Could you check a few things on this drawing? It's one solid part, dimensions in mm from its lowest x, y, z. A direction names the side the tool comes from. Give positions to 0.01 mm unless a question says otherwise; leave off trailing zeros. Loops run counter-clockwise (first coordinate to the right, second up) from the corner with the lowest first, then second, coordinate; pieces in that order, holes last. Notation, with made-up numbers: M 57,-29.75 L 75,-29.75 A18 cw 75,-13.75 Z; hole C 77,-39 d5. An arc over 180 degrees is marked long. Answer as CSV lines item,"result". Start each with the question number.
Item 1: If I drill on line 1 along X through (y, z) = (49, 3.5); line 2 along X through (y, z) = (20, 29.5); line 3 along X through (y, z) = (6.5, 3), over which ranges is the centre line in solid material (lowest first)? Write a range as from..to.
Item 2: For the marked faces 1, 2, 3, 4 and 5, which set-ups out of +Z, -Z, +X, -X, +Y, -Y let a thin tool reach every point of the face, with its end or its side?
Item 3: Will these pins go through, and if not, where does the flat tip stop? P1, Ø3, axis at y = 30.5, z = 32, coming from the +X side; P2, Ø0.8, axis at x = 32.5, z = 67, coming from the -Y side; P3, Ø3, axis at x = 39.45, z = 37.92, coming from the -Y side; P4, Ø1.5, axis at y = 33.5, z = 41.5, coming from the -X side.
Item 4: If we mould it in two halves opening along Z, with no side actions, what happens to the marked faces 6, 7 and 8? For each: released by +Z, released by -Z, zero draft, split by the parting line, or undercut.
Item 5: I want a section at B-B on z = 35. List the corners of the cut face in (x, y) for me.
Item 6: I want a section at A-A on x = 33. List the corners of the cut face in (y, z) for me, plus the area to 3 significant figures.
Item 7: I want a section at C-C on x = 45.5. List the corners of the cut face in (y, z) for me.
Item 8: I want a section at D-D on y = 26. List the corners of the cut face in (x, z) for me.
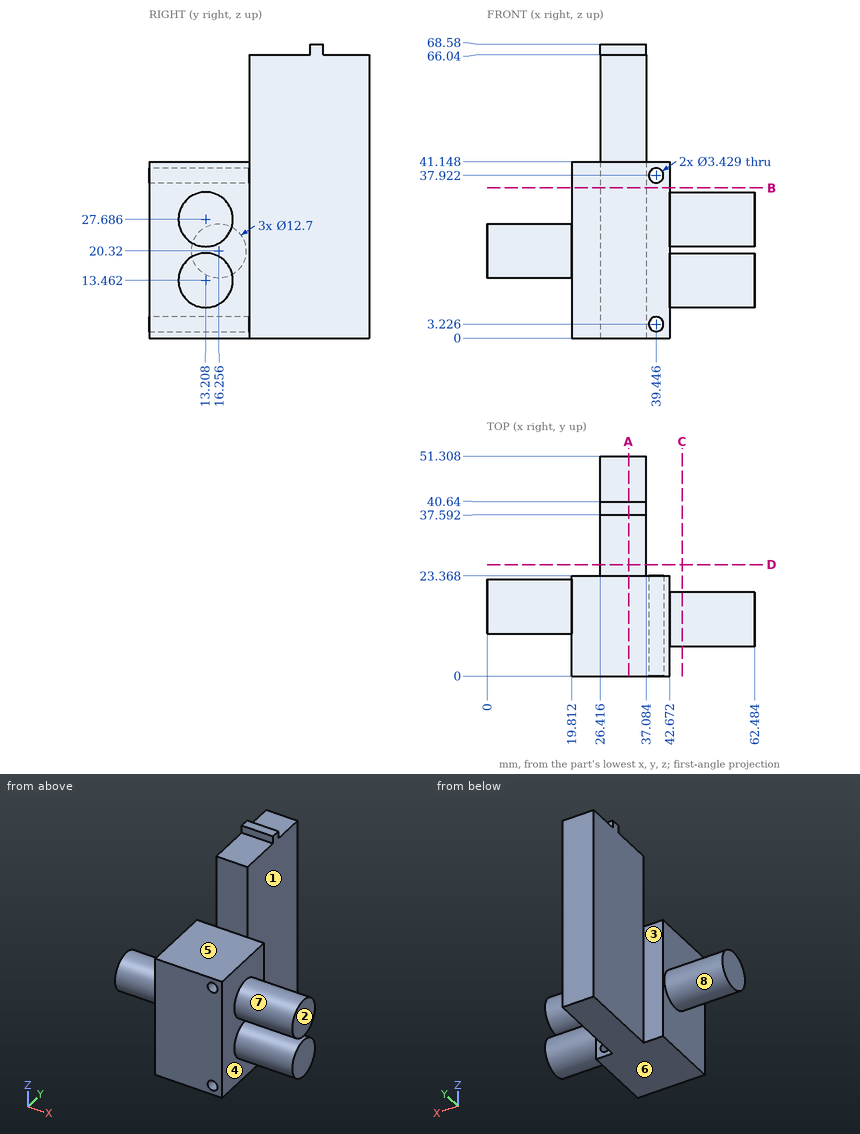
Result:
1,line 1,"26.42..37.08"
1,line 2,"19.81..42.67"
1,line 3,"19.81..37.75, 41.15..42.67"
2,face 1,"+Z, -Z, +X, +Y"
2,face 2,"+Z, -Z, +X, +Y, -Y"
2,face 3,"+Z, -Z, -X, +Y"
2,face 4,"+X"
2,face 5,"+Z, +X, -X, -Y"
3,P1,"x = 37.08"
3,P2,"y = 37.59"
3,P3,"through"
3,P4,"x = 26.42"
4,face 6,"released by -Z"
4,face 7,"undercut"
4,face 8,"split by the parting line"
5,outline,"M 19.81,0 L 42.67,0 L 42.67,23.37 L 37.08,23.37 L 37.08,51.31 L 26.42,51.31 L 26.42,23.37 L 19.81,23.37 Z"
6,outline,"M 0,0 L 51.31,0 L 51.31,66.04 L 40.64,66.04 L 40.64,68.58 L 37.59,68.58 L 37.59,66.04 L 23.37,66.04 L 23.37,41.15 L 0,41.15 Z"
6,area,"2,810 mm^2"
7,outline,"C 13.21,13.46 d12.7; C 13.21,27.69 d12.7"
8,outline,"M 26.42,0 L 37.08,0 L 37.08,66.04 L 26.42,66.04 Z"
